```python
from build123d import *

# Parameters (mm, degrees)
SKETCH7_R          = 20
CUT_EXTRUDE1_DEPTH = 121.438221623


with BuildPart() as part:
    # Sketch6 → Revolve2 (revolve)
    with BuildSketch(Plane.XY, mode=Mode.PRIVATE) as revolve2_sk:
        Polygon((85, 0), (61.011931512, 0), (54.658752463, -5.575845989), (0.011931512, -5.575845989), (0.011931512, -7.575845989), (55.411931512, -7.575845989), (61.76511056, -2), (85, -2), align=None)
    revolve(revolve2_sk.sketch.rotate(Axis((0.011931512, 83.769679303, 0), (0, -1, 0)), 180), axis=Axis((0.011931512, 83.769679303, 0), (0, -1, 0)))

    # Sketch7 → Cut-Extrude1 (cut, through all)
    with BuildSketch(Plane.XZ.offset(7.575845989)):
        Circle(SKETCH7_R)
    extrude(amount=-CUT_EXTRUDE1_DEPTH, mode=Mode.SUBTRACT)


solid = part.part
```
The model under review builds one solid part; all positions refer to its coordinate system, in mm. A direction names the side the tool comes from. Round coordinates to 2 decimals unless told otherwise and drop trailing zeros. Loops run counter-clockwise (first coordinate to the right, second up) from the corner with the lowest first, then second, coordinate; pieces in that order, holes last. Notation, with made-up numbers: M 41,-30 L 69,-30 A27 ccw 69,5 Z; hole C 30.25,-21 d8. An arc over 180 degrees is marked long. Put each result on its own line as item: value.
Q1. Machinability: for faces 1 (the cylindrical face through (-81.05, -0.99, -25.53)), 2 (the flat face through (-24, -5.576, -1)), 3 (the flat face through (44, -2, -44)), which of the approach directions +Z, -Z, +X, -X, +Y, -Y give a long, thin tool a straight path to every point of the face, cutting with its end or side? Answer none if there is none.
Result set:
face 1: +Y, -Y
face 2: +Y
face 3: -Y
Q2. Mouldability with a two-part tool opening along Z and no side actions: class faces 4 (the conical face through (-25.735, -7.227, 49.502)), 5 (the flat face through (58, 0, -20)), 6 (the conical face through (54.91, -5.31, -2.42)) as released by +Z, released by -Z, zero draft, split by the parting line, or undercut.
Result set:
face 4: split by the parting line
face 5: zero draft
face 6: undercut
Q3. Consider section B-B, the plane y = -3.25. Give the boundary of the cut face in (x, z), then the cut area to 3 significant figures.
Result set:
outline: C 0.01,0 d120.66; hole C 0.01,0 d114.59
area: 1,120 mm²
Q4. To check wall thickness, follow L1, parallel to Y at x = 24.5, z = -76.5; L2, parallel to Y at x = -14.5, z = -37; L3, parallel to Z at x = 0, y = -6.2. State the ranges of each line that lie inside material, in increasing order.
Result set:
L1: y = -2 to 0
L2: y = -7.58 to -5.58
L3: z = -56.97 to -20, 20 to 56.97
Q5. Consider section A-A, the plane z = 0. Give the boundary of the cut face in (x, y), then the cut area to 3 significant figures.
Result set:
outline: M -84.98,-2 L -61.74,-2 L -55.39,-7.58 L -20,-7.58 L -20,-5.58 L -54.63,-5.58 L -60.99,0 L -84.98,0 Z; M 20,-7.58 L 55.41,-7.58 L 61.77,-2 L 85,-2 L 85,0 L 61.01,0 L 54.66,-5.58 L 20,-5.58 Z
area: 268 mm²
Q6. Consider section C-C, the plane x = -72.5. Give the boundary of the cut face in (y, z).
Result set:
outline: M -2,-44.33 L 0,-44.33 L 0,44.33 L -2,44.33 Z
Q7. For pin 1 (8 mm diameter, centred on x = 27, z = -50, fed in from +Y); pin 2 (4 mm diameter, centred on x = -3.5, y = -5.5, fed in from -Z); pin 3 (4 mm diameter, centred on y = -1.5, z = -35.5, fed in from +X), all flat-tipped, find the tip position at first contact; note any pin that passes through.
Result set:
pin 1: stops at y = -0.16
pin 2: stops at z = -59.94
pin 3: stops at x = 78.12
